```python
from build123d import *

# Parameters (mm, degrees)
SKETCH2_W                                      = 80
SKETCH2_H                                      = 40
BOSS_EXTRUDE1_DEPTH                            = 3.175
M4_CLEARANCE_HOLE1_D                           = 4.3
CSK_FOR_M4_FLAT_HEAD_MACHINE_SCREW2_AT_2_COUNT = 2
CSK_FOR_M4_FLAT_HEAD_MACHINE_SCREW2_AT_2_PITCH = 16
CSK_FOR_M4_FLAT_HEAD_MACHINE_SCREW2_AT_3_COUNT = 2
CSK_FOR_M4_FLAT_HEAD_MACHINE_SCREW2_AT_3_PITCH = 22.627416998
CSK_FOR_M4_FLAT_HEAD_MACHINE_SCREW2_AT_4_COUNT = 2
CSK_FOR_M4_FLAT_HEAD_MACHINE_SCREW2_AT_4_PITCH = 16


with BuildPart() as part:
    # Sketch2 → Boss-Extrude1 (new body)
    with BuildSketch(Plane(origin=(0, 0, 0), x_dir=(1, 0, 0), z_dir=(0, 1, 0))):
        Rectangle(SKETCH2_W, SKETCH2_H)
    extrude(amount=BOSS_EXTRUDE1_DEPTH)

    # M4 Clearance Hole1 (through all)
    with Locations(Plane(origin=(0, 3.175, 0), x_dir=(1, 0, 0), z_dir=(0, 1, 0))):
        with Locations((-35, 10), (35, 10), (35, -10), (-35, -10)):
            Hole(M4_CLEARANCE_HOLE1_D / 2)

    # Sketch6 → CSK for M4 Flat Head Machine Screw2 (revolve, cut)
    with BuildSketch(Plane(origin=(-8, 3.175, -8), x_dir=(0, 0, 1), z_dir=(1, 0, 0))):
        Polygon((0, 0), (0, 3.175), (2.15, 3.175), (2.15, 2.55), (4.7, 0), align=None)
    csk_for_m4_flat_head_machine_screw2 = revolve(axis=Axis((-8, 9.525, -8), (0, -1, 0)), mode=Mode.SUBTRACT)

    # CSK for M4 Flat Head Machine Screw2 at 2: CSK for M4 Flat Head Machine Screw2 ×2
    with Locations(*[(i * CSK_FOR_M4_FLAT_HEAD_MACHINE_SCREW2_AT_2_PITCH, 0, 0) for i in range(1, CSK_FOR_M4_FLAT_HEAD_MACHINE_SCREW2_AT_2_COUNT)]):
        add(csk_for_m4_flat_head_machine_screw2, mode=Mode.SUBTRACT)

    # CSK for M4 Flat Head Machine Screw2 at 3: CSK for M4 Flat Head Machine Screw2 ×2
    with Locations(*[Vector(0.707106781186545, 0, 0.70710678118655) * (i * CSK_FOR_M4_FLAT_HEAD_MACHINE_SCREW2_AT_3_PITCH) for i in range(1, CSK_FOR_M4_FLAT_HEAD_MACHINE_SCREW2_AT_3_COUNT)]):
        add(csk_for_m4_flat_head_machine_screw2, mode=Mode.SUBTRACT)

    # CSK for M4 Flat Head Machine Screw2 at 4: CSK for M4 Flat Head Machine Screw2 ×2
    with Locations(*[(0, 0, i * CSK_FOR_M4_FLAT_HEAD_MACHINE_SCREW2_AT_4_PITCH) for i in range(1, CSK_FOR_M4_FLAT_HEAD_MACHINE_SCREW2_AT_4_COUNT)]):
        add(csk_for_m4_flat_head_machine_screw2, mode=Mode.SUBTRACT)


solid = part.part
```
Input: part model. Units: mm. Frame: model coordinates. Coordinates: 2 decimals unless noted, no trailing zeros. Loops run counter-clockwise (first coordinate to the right, second up) from the corner with the lowest first, then second, coordinate; pieces in that order, holes last.
Q1. Contact query for a flat-ended pin moving along its axis: pin 1 (7 mm diameter, centred on x = -8, z = 8, fed in from +Y) (3 decimals). Output: stop coordinate, or through.
Results are:
pin 1: stops at y = 1.975
Q2. Mould query, pull axis Z, two halves, no side actions, for faces 1 (the flat face through (-1, 2, 20)), 2 (the cylindrical face through (6.19, 0.32, 9.16)), 3 (the flat face through (-1, 2, -20)), 4 (the flat face through (40, 2, 0)). Classes: +Z half, -Z half, draft (parallel to the pull), parting line (faces both ways), or undercut.
Results are:
face 1: +Z half
face 2: undercut
face 3: -Z half
face 4: draft
Q3. Line query: line 1 along Z through (x, y) = (35, 2.55); line 2 along Z through (x, y) = (-8, 0.45); line 3 along X through (y, z) = (2.45, -10). Output: solid intervals per line, ascending.
Results are:
line 1: z = -20 to -12.15, -7.85 to 7.85, 12.15 to 20
line 2: z = -20 to -10.15, -5.85 to 5.85, 10.15 to 20
line 3: x = -40 to -37.15, -32.85 to -11.44, -4.56 to 4.56, 11.44 to 32.85, 37.15 to 40
Q4. Section A-A, the plane x = -35. Return the cut outline in (y, z) (3 decimals), and give its area (3 significant figures).
Results are:
outline: (0, -20) - (3.175, -20) - (3.175, -12.15) - (0, -12.15) - close; (0, -7.85) - (3.175, -7.85) - (3.175, 7.85) - (0, 7.85) - close; (0, 12.15) - (3.175, 12.15) - (3.175, 20) - (0, 20) - close
area: 99.7 mm2
Q5. Section C-C, the plane x = -8. Return the cut outline in (y, z) (3 decimals), and give its area (3 significant figures).
Results are:
outline: (0, -20) - (3.175, -20) - (3.175, -12.7) - (0.625, -10.15) - (0, -10.15) - close; (0, -5.85) - (0.625, -5.85) - (3.175, -3.3) - (3.175, 3.3) - (0.625, 5.85) - (0, 5.85) - close; (0, 10.15) - (0.625, 10.15) - (3.175, 12.7) - (3.175, 20) - (0, 20) - close
area: 86.7 mm2
Q6. Section B-B, the plane y = 2.4. Give the number of separate pieces and of enclosed holes in the cut face, and give its area (3 significant figures).
Results are:
separate pieces: 1
enclosed holes: 8
area: 2,950 mm2
